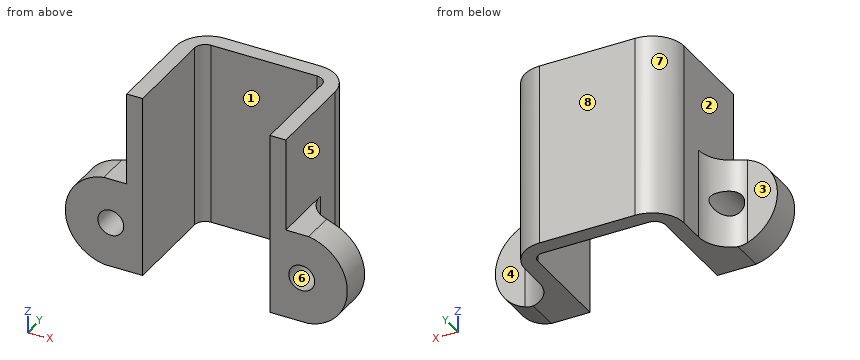
```python
from build123d import *

# Parameters (mm, degrees)
EXTRUDE1_DEPTH            = 17.3
SKETCH2_W                 = 5.8
SKETCH2_H                 = 8.5
EXTRUDE2_DEPTH            = 8.8
SKETCH3_R                 = 1
EXTRUDE3_DEPTH            = 5
F_2_CLEARANCE_HOLE1_D     = 2.4384
F_2_CLEARANCE_HOLE1_DEPTH = 11.5


with BuildPart() as part:
    # Sketch1 → Extrude1 (new body)
    with BuildSketch(Plane.XY):
        with BuildLine():
            Line((-13.3, 0), (-6, 0))
            Line((-6, 0), (-6, 9))
            ThreePointArc((-6, 9), (-5.707106781, 9.707106781), (-5, 10))
            Line((-5, 10), (5, 10))
            ThreePointArc((5, 10), (5.707106781, 9.707106781), (6, 9))
            Line((6, 9), (6, 0))
            Line((6, 0), (13.3, 0))
            Line((13.3, 0), (13.3, 3))
            Line((13.3, 3), (10.5, 3))
            ThreePointArc((10.5, 3), (8.378679656, 3.878679656), (7.5, 6))
            Line((7.5, 6), (7.5, 8.5))
            ThreePointArc((7.5, 8.5), (6.621320344, 10.621320344), (4.5, 11.5))
            Line((4.5, 11.5), (-4.5, 11.5))
            ThreePointArc((-4.5, 11.5), (-6.621320344, 10.621320344), (-7.5, 8.5))
            Line((-7.5, 8.5), (-7.5, 6))
            ThreePointArc((-7.5, 6), (-8.378679656, 3.878679656), (-10.5, 3))
            Line((-10.5, 3), (-13.3, 3))
            Line((-13.3, 3), (-13.3, 0))
        make_face()
    extrude(amount=EXTRUDE1_DEPTH)

    # Sketch2 → Extrude2 (cut)
    with BuildSketch(Plane.XY.offset(17.3)):
        with Locations((-10.4, 4.25)):
            Rectangle(SKETCH2_W, SKETCH2_H)
        with Locations((10.4, 4.25)):
            Rectangle(SKETCH2_W, SKETCH2_H)
    extrude(amount=-EXTRUDE2_DEPTH, mode=Mode.SUBTRACT)

    # Sketch3 → Extrude3 (cut)
    with BuildSketch(Plane.XZ):
        with Locations(Location((-9, 4.25, 0), (0, 0, 270))):  # turned: the seam where the file's is
            Circle(SKETCH3_R)
        with Locations(Location((9, 4.25, 0), (0, 0, 270))):  # turned: the seam where the file's is
            Circle(SKETCH3_R)
        with BuildLine():
            Line((9.653834842, 8.5), (9.653834842, 9.262963398))
            Line((9.653834842, 9.262963398), (15.079268599, 9.262963398))
            Line((15.079268599, 9.262963398), (15.079268599, -0.486230121))
            Line((15.079268599, -0.486230121), (9.653834842, -0.486230121))
            Line((9.653834842, -0.486230121), (9.653834842, 0))
            ThreePointArc((9.653834842, 0), (13.3, 4.25), (9.653834842, 8.5))
        make_face()
        with BuildLine():
            Line((-9.653834842, -0.486230121), (-9.653834842, 0))
            ThreePointArc((-9.653834842, 0), (-13.3, 4.25), (-9.653834842, 8.5))
            Line((-9.653834842, 8.5), (-9.653834842, 9.262963398))
            Line((-9.653834842, 9.262963398), (-15.079268599, 9.262963398))
            Line((-15.079268599, 9.262963398), (-15.079268599, -0.486230121))
            Line((-15.079268599, -0.486230121), (-9.653834842, -0.486230121))
        make_face()
    extrude(amount=-EXTRUDE3_DEPTH, mode=Mode.SUBTRACT)

    # #2 Clearance Hole1
    with Locations(Plane(origin=(-9, 0, 4.25), x_dir=(0, 0, -1), z_dir=(0, -1, 0))):
        with Locations((0, 0), (0, 18)):
            Hole(F_2_CLEARANCE_HOLE1_D / 2, depth=F_2_CLEARANCE_HOLE1_DEPTH)


solid = part.part
```
Geometry: final body of the model. Coordinates: model frame, mm. Face numbers are marked on the shaded views. A direction names the side the tool comes from. Round coordinates to 2 decimals unless told otherwise and drop trailing zeros. Order: outer loops, then holes, each group sorted by start corner. A loop starts at its lowest first (then second) coordinate and runs counter-clockwise, first axis right, second up. Notation, with made-up numbers: (-14, 29) - (20, 29) arc R15 ccw to (20, 56) - close; hole circle Ø1 at (-38.5, 39). An arc over 180 degrees is marked (long way). Write item = value, one per line. Start each with the question number.
Q1. Pull-direction query (X, two-part tool) for the marked faces 6, 7 and 8; classes: +X half, -X half, draft (parallel to the pull), parting line (faces both ways), or undercut.
Q2. Cut plane B-B on z = 15.5. Return the cut outline in (x, y), and give its area (3 significant figures).
Q3. Cut plane C-C on x = -9. Return the cut outline in (y, z), and give its area (3 significant figures).
Q4. Cut plane A-A on y = 2.5. Return the cut outline in (x, z).
Q5. Ray query, line 1 (X direction, y = 1.3, z = 4.25); line 2 (Z direction, x = 9, y = 1.7); line 3 (X direction, y = 1.5, z = 12.75). Return the intervals inside material, ascending. Write a range as from..to.
Q6. Cut plane D-D on z = 4.25. Return the cut outline in (x, y), and give its area (3 significant figures).
Q7. Access query for the marked faces 1, 2, 3, 4 and 5. Directions: +Z, -Z, +X, -X, +Y, -Y. A direction counts if a zero-diameter tool reaches every point of the face in a straight line with its end or side. Return the directions, or none.
Q8. Pin query (flat end, axial travel): pin 1 (2 mm diameter, centred on x = 9, z = 4.25, fed in from +Y); pin 2 (8 mm diameter, centred on x = 1, z = 8.5, fed in from -Y); pin 3 (1.7 mm diameter, centred on x = -9, y = 2.5, fed in from +Z); pin 4 (3 mm diameter, centred on x = -12.5, z = 4, fed in from +Y). Return the tip coordinate at first contact, or that it passes through.
Outcome:
q1.face_6 = undercut
q1.face_7 = -X half
q1.face_8 = draft
q2.outline = (-7.5, 0) - (-6, 0) - (-6, 9) arc R1 cw to (-5, 10) - (5, 10) arc R1 cw to (6, 9) - (6, 0) - (7.5, 0) - (7.5, 8.5) arc R3 ccw to (4.5, 11.5) - (-4.5, 11.5) arc R3 ccw to (-7.5, 8.5) - close
q2.area = 49.1 mm^2
q3.outline = (0, 0) - (3.4, 0) - (3.4, 3.03) - (0, 3.03) - close; (0, 5.47) - (3.4, 5.47) - (3.4, 8.5) - (0, 8.5) - close
q3.area = 20.6 mm^2
q4.outline = (-9.65, 0) - (-6, 0) - (-6, 17.3) - (-7.5, 17.3) - (-7.5, 8.5) - (-9.65, 8.5) arc R4.3 ccw to start; (6, 0) - (9.65, 0) arc R4.3 ccw to (9.65, 8.5) - (7.5, 8.5) - (7.5, 17.3) - (6, 17.3) - close; hole circle Ø2.44 at (-9, 4.25); hole circle Ø2.44 at (9, 4.25)
q5.line_1 = -13.3..-10.22, -7.78..-6, 6..7.78, 10.22..13.3
q5.line_2 = 0..3.03, 5.47..8.5
q5.line_3 = -7.5..-6, 6..7.5
q6.outline = (-13.3, 0) - (-10.22, 0) - (-10.22, 3.01) arc R3 cw to (-10.5, 3) - (-13.3, 3) - close; (-7.78, 0) - (-6, 0) - (-6, 9) arc R1 cw to (-5, 10) - (5, 10) arc R1 cw to (6, 9) - (6, 0) - (7.78, 0) - (7.78, 4.73) arc R3 cw to (7.5, 6) - (7.5, 8.5) arc R3 ccw to (4.5, 11.5) - (-4.5, 11.5) arc R3 ccw to (-7.5, 8.5) - (-7.5, 6) arc R3 cw to (-7.78, 4.73) - close; (10.22, 0) - (13.3, 0) - (13.3, 3) - (10.5, 3) arc R3 cw to (10.22, 3.01) - close
q6.area = 70.4 mm^2
q7.face_1 = +Z, -Z, -Y
q7.face_2 = +Z, -X, +Y
q7.face_3 = +Z, -Z, -X, +Y
q7.face_4 = +Z, -Z, +X, +Y
q7.face_5 = +Z, +X, +Y
q8.pin_1 = through
q8.pin_2 = 10
q8.pin_3 = 8.5
q8.pin_4 = 3
